```python
from build123d import *

# Parameters (mm, degrees)
SKETCH1_R          = 34.925
EXTRUDE1_DEPTH     = 12.7
SKETCH3_R          = 3.3655
CUT_EXTRUDE2_DEPTH = 12.7
CIRPATTERN1_COUNT  = 6
SKETCH5_R          = 9.525
EXTRUDE2_DEPTH     = 129.54
EXTRUDE3_START     = 50.8
SKETCH6_R          = 9.525
EXTRUDE3_DEPTH     = 50.8


with BuildPart() as part:
    # Sketch1 → Extrude1 (new body)
    with BuildSketch(Plane(origin=(0, 0, 0), x_dir=(1, 0, 0), z_dir=(0, 1, 0))):
        with Locations(Location((0, 0, 0), (0, 0, 270))):
            Circle(SKETCH1_R)
    extrude(amount=EXTRUDE1_DEPTH)

    # Sketch3 → Cut-Extrude2 (cut)
    with BuildSketch(Plane(origin=(0, 0, 0), x_dir=(1, 0, 0), z_dir=(0, 1, 0))):
        with Locations(Location((0, 29.337, 0), (0, 0, 270))):
            Circle(SKETCH3_R)
    cut_extrude2 = extrude(amount=CUT_EXTRUDE2_DEPTH, mode=Mode.SUBTRACT)

    # CirPattern1: Cut-Extrude2 ×6 about axis
    cirpattern1_axis = Axis((0, 0, 0), (0, 1, 0))
    for i in range(1, CIRPATTERN1_COUNT):
        add(cut_extrude2.rotate(cirpattern1_axis, i * 360 / CIRPATTERN1_COUNT), mode=Mode.SUBTRACT)

    # Sketch5 → Extrude2 (add)
    with BuildSketch(Plane(origin=(0, 0, 0), x_dir=(1, 0, 0), z_dir=(0, 1, 0))):
        with Locations(Location((0, 0, 0), (0, 0, 270))):
            Circle(SKETCH5_R)
    extrude(amount=-EXTRUDE2_DEPTH)

    # Sketch6 → Extrude3 (add)
    with BuildSketch(Plane(origin=(0, 12.7, 0), x_dir=(-1, 0, 0), z_dir=(0, 1, 0)).offset(EXTRUDE3_START)):
        with Locations(Location((0, 0, 0), (0, 0, 90))):
            Circle(SKETCH6_R)
    extrude(amount=-EXTRUDE3_DEPTH)


solid = part.part
```
Here's how the part is built. I have some questions about the finished solid (model axes, mm). A direction names the side the tool comes from. Round coordinates to 2 decimals unless told otherwise and drop trailing zeros. Write each loop counter-clockwise with the first axis right and the second up, starting at its lowest first coordinate (ties: lowest second). Pieces come first, ordered by that corner, then holes.
Q1. If we section it at C-C on y = -83: Write out the boundary of the cut face in (x, z) (3 decimals), plus the area to 3 significant figures.
Q2. Please list where these lines run through material, in increasing order: probe 1 along Y at (x, z) = (-6, -10); probe 2 along X at (y, z) = (3.5, 28); probe 3 along X at (y, z) = (-26, -0.5).
Q3. If we section it at D-D on x = -17.5: Write out the boundary of the cut face in (y, z), plus the area to 3 significant figures.
Q4. Which directions (+Z, -Z, +X, -X, +Y, -Y) give clear straight access to the entire face, cutting with the end or side of a thin tool? Please do faces 4 (the cylindrical face through (-28.392, 6.261, 16.221)), 5 (the flat face through (-7, 0, 7)), 6 (the flat face through (-7, 12.7, 7)).
Q5. If we section it at A-A on x = 0: Write out the boundary of the cut face in (y, z) (1 decimal).
Q6. If we mould it in two halves opening along X, with no side actions, what happens to faces 1 (the cylindrical face through (-5.796, 38.456, -7.559)), 2 (the cylindrical face through (22.42, 6.26, 16.22)), 3 (the flat face through (0, -129.54, 0))? For each: +X half, -X half, draft (parallel to the pull), parting line (faces both ways), or undercut.
Q7. If we section it at B-B on z = 0: Write out the boundary of the cut face in (x, y) (3 decimals).
Q8. Will these pins go through, and if not, where does the flat tip stop? P1, Ø11, axis at x = 25.41, z = 14.67, coming from the -Y side; P2, Ø12, axis at y = -86, z = 12.5, coming from the -X side; P3, Ø9, axis at x = 25.41, z = -14.67, coming from the +Y side; P4, Ø6, axis at y = -50, z = 13.5, coming from the -X side.
Answer below:
1. outline: circle Ø19.05 at (0, 0)
1. area: 285 mm2
2. probe 1: y = 0 to 12.7
2. probe 2: x = -20.87 to -3.09, 3.09 to 20.87
2. probe 3: x = -9.51 to 9.51
3. outline: (0, -30.22) - (12.7, -30.22) - (12.7, 30.22) - (0, 30.22) - close
3. area: 768 mm2
4. face 4: +Y, -Y
4. face 5: -Y
4. face 6: +Y
5. outline: (-129.5, -9.5) - (0, -9.5) - (0, -26) - (12.7, -26) - (12.7, -9.5) - (63.5, -9.5) - (63.5, 9.5) - (12.7, 9.5) - (12.7, 26) - (0, 26) - (0, 9.5) - (-129.5, 9.5) - close; (0, -34.9) - (12.7, -34.9) - (12.7, -32.7) - (0, -32.7) - close; (0, 32.7) - (12.7, 32.7) - (12.7, 34.9) - (0, 34.9) - close
6. face 1: parting line
6. face 2: undercut
6. face 3: draft
7. outline: (-34.925, 0) - (-9.525, 0) - (-9.525, -129.54) - (9.525, -129.54) - (9.525, 0) - (34.925, 0) - (34.925, 12.7) - (9.525, 12.7) - (9.525, 63.5) - (-9.525, 63.5) - (-9.525, 12.7) - (-34.925, 12.7) - close
8. P1: stops at y = 0
8. P2: stops at x = -6.96
8. P3: stops at y = 12.7
8. P4: passes through
